Verification items for the finished model (mm, model axes). A direction names the side the tool comes from. Coordinates: 2 decimals unless noted, no trailing zeros. Loops run counter-clockwise (first coordinate to the right, second up) from the corner with the lowest first, then second, coordinate; pieces in that order, holes last. Notation, with made-up numbers: (-17, 83.25) -> (-12, 83.25) arc R16 cw to (-12, 97.25) -> close; hole circle Ø11 at (68, 86). An arc over 180 degrees is marked (long way). Write item = value, one per line.
```python
from build123d import *

# Parameters (mm, degrees)
SKETCH1_R           = 10
BOSS_EXTRUDE1_DEPTH = 63.25
SKETCH2_R           = 12.5
BOSS_EXTRUDE2_DEPTH = 6.43
SKETCH3_R           = 4
CUT_EXTRUDE1_DEPTH  = 66.673910345


with BuildPart() as part:
    # Sketch1 → Boss-Extrude1 (new body)
    with BuildSketch(Plane(origin=(0, 0, 0), x_dir=(0, 0, -1), z_dir=(1, 0, 0))):
        Circle(SKETCH1_R)
    extrude(amount=BOSS_EXTRUDE1_DEPTH)

    # Sketch2 → Boss-Extrude2 (add)
    with BuildSketch(Plane.ZY):
        Circle(SKETCH2_R)
    extrude(amount=-BOSS_EXTRUDE2_DEPTH)

    # Sketch3 → Cut-Extrude1 (cut, through all)
    with BuildSketch(Plane(origin=(63.25, 0, 0), x_dir=(0, 0, -1), z_dir=(1, 0, 0))):
        Circle(SKETCH3_R)
    extrude(amount=-CUT_EXTRUDE1_DEPTH, mode=Mode.SUBTRACT)


solid = part.part
```
1) Release check for a two-part mould opening along Z. For faces 1 (the face through (3.17, 3.755, 11.923)), 2 (the face through (6.43, 10.2, -0.1)), 3 (the face through (32.068, -3.905, 0.867)) record: pulls with the +Z half, pulls with the -Z half, needs draft (parallel to the pull), parting line crosses it, or undercut.
Ans:
face_1 = parting line crosses it
face_2 = needs draft
face_3 = undercut
2) Sectioned sample at D-D, the plane z = 4.75. Record the cut outline in (x, y), plus the area to 3 significant figures.
Ans:
outline = (0, -11.56) -> (6.43, -11.56) -> (6.43, -8.8) -> (63.25, -8.8) -> (63.25, 8.8) -> (6.43, 8.8) -> (6.43, 11.56) -> (0, 11.56) -> close
area = 1,150 mm2
3) Sectioned sample at C-C, the plane x = 17. Record the cut outline in (y, z).
Ans:
outline = circle Ø20 at (0, 0); hole circle Ø8 at (0, 0)
4) Sectioned sample at A-A, the plane y = 0. Record the cut outline in (x, z).
Ans:
outline = (0, -12.5) -> (6.43, -12.5) -> (6.43, -10) -> (63.25, -10) -> (63.25, -4) -> (0, -4) -> close; (0, 4) -> (63.25, 4) -> (63.25, 10) -> (6.43, 10) -> (6.43, 12.5) -> (0, 12.5) -> close
5) Material ranges on line 1 (Y direction, x = 48, z = 0); line 2 (Y direction, x = 4, z = 0); line 3 (X direction, y = 5, z = 9.5), recorded low to high.
Ans:
line_1 = -10 to -4, 4 to 10
line_2 = -12.5 to -4, 4 to 12.5
line_3 = 0 to 6.43
6) Tool access check on faces 4 (the face through (34.44, -9.76, 2.17)), 5 (the face through (63.25, -4.3, 0.1)). Record the directions out of +Z, -Z, +X, -X, +Y, -Y that give a thin tool (end or side, any length) a straight path to the whole face; none if there is none.
Ans:
face_4 = +X
face_5 = +Z, -Z, +X, +Y, -Y
7) Depth check by flat-ended pin: pin 1 Ø6 at (x, z) = (16.5, -3.5) entering from -Y; pin 2 Ø6 at (x, y) = (46.5, -5) entering from +Z; pin 3 Ø10 at (x, y) = (43, -6.5) entering from -Z; pin 4 Ø7 at (y, z) = (0, 0) entering from -X. Enter the tip coordinate at first touch or a pass-through.
Ans:
pin_1 = -9.99
pin_2 = 9.8
pin_3 = -9.89
pin_4 = through
